Could you check a few things on this drawing? It's one solid part, dimensions in mm from its lowest x, y, z. A direction names the side the tool comes from. Give positions to 0.01 mm unless a question says otherwise; leave off trailing zeros. Order: outer loops, then holes, each group sorted by start corner. A loop starts at its lowest first (then second) coordinate and runs counter-clockwise, first axis right, second up. Notation, with made-up numbers: M 26,1.25 L 82,1.25 A20 ccw 82,11.25 Z; hole C -39,-16 d10. An arc over 180 degrees is marked long. Use one line per item in the form item = value.
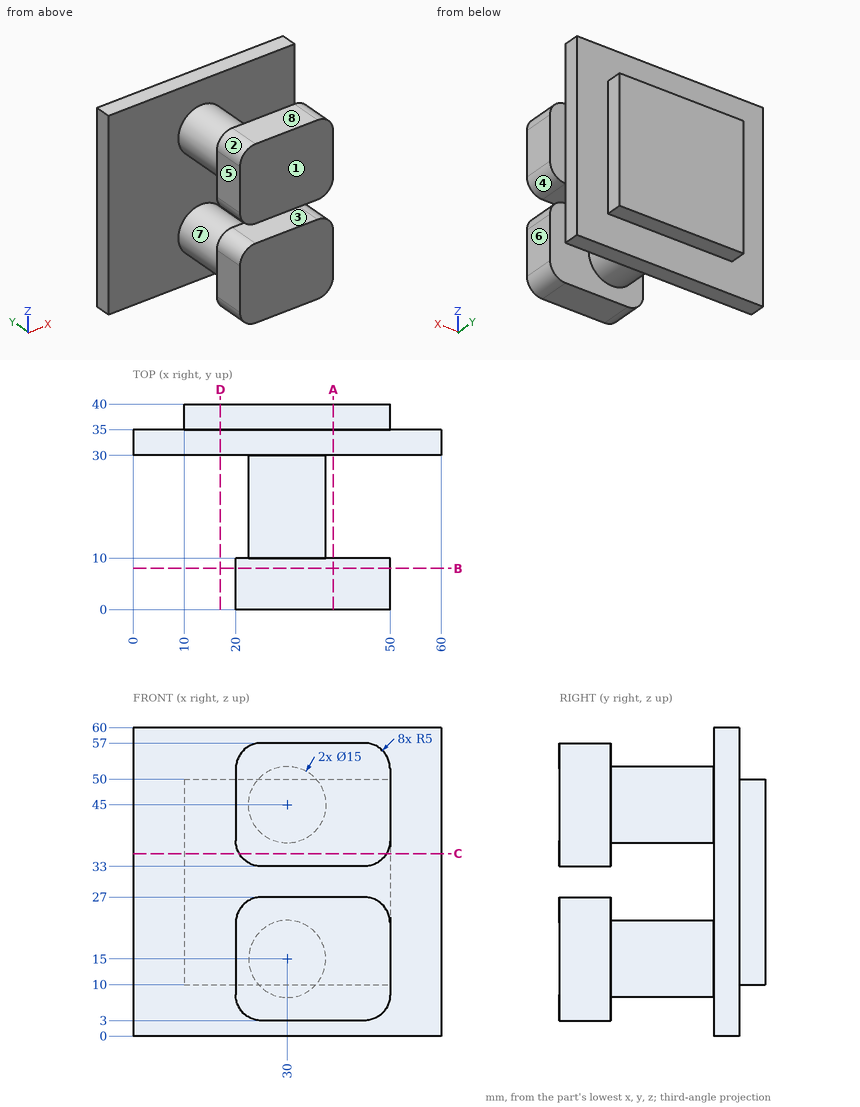
Q1. I want a section at B-B on y = 8. Write out the boundary of the cut face in (x, z), then the cut area to 3 significant figures.
Found:
outline = M 20,8 A5 ccw 25,3 L 45,3 A5 ccw 50,8 L 50,22 A5 ccw 45,27 L 25,27 A5 ccw 20,22 Z; M 20,38 A5 ccw 25,33 L 45,33 A5 ccw 50,38 L 50,52 A5 ccw 45,57 L 25,57 A5 ccw 20,52 Z
area = 1,400 mm²
Q2. I'm going to push flat-ended pins straight in: pin 1 Ø11 at (y, z) = (3.5, 41.5) entering from -X; pin 2 Ø2 at (y, z) = (22.5, 11.5) entering from -X; pin 3 Ø5 at (x, y) = (34, 4.5) entering from +Z. Where does each tip first touch, or does it pass through?
Found:
pin_1 = 20
pin_2 = 22.93
pin_3 = 57
Q3. I want a section at C-C on z = 35.5. Write out the boundary of the cut face in (x, y), then the cut area to 3 significant figures.
Found:
outline = M 0,30 L 60,30 L 60,35 L 50,35 L 50,40 L 10,40 L 10,35 L 0,35 Z; M 20.67,0 L 49.33,0 L 49.33,10 L 20.67,10 Z
area = 787 mm²
Q4. I need wall thicknesses on L1, parallel to Z at x = 44.5, y = 5.5; L2, parallel to Y at x = 42.5, z = 21.5; L3, parallel to Y at x = 43.5, z = 3.5. Which ranges of each line are inside material? Lowest first, please.
Found:
L1 = 3 to 27, 33 to 57
L2 = 0 to 10, 30 to 40
L3 = 0 to 10, 30 to 35
Q5. On a 3-axis mill with a long thin cutter (end or side, diameter ignored), from which of +Z, -Z, +X, -X, +Y, -Y can I reach the whole of each face in a straight line? I mean the marked faces 5, 6, 7 and 8. Say none if no direction works.
Found:
face_5 = +Z, -Z, -X, -Y
face_6 = +Z, -Z, +X, -Y
face_7 = none
face_8 = +Z, +X, -X, -Y
Q6. I want a section at D-D on x = 17. Write out the boundary of the cut face in (y, z), then the cut area to 3 significant figures.
Found:
outline = M 30,0 L 35,0 L 35,10 L 40,10 L 40,50 L 35,50 L 35,60 L 30,60 Z
area = 500 mm²
Q7. I want a section at A-A on x = 39. Write out the boundary of the cut face in (y, z).
Found:
outline = M 0,3 L 10,3 L 10,27 L 0,27 Z; M 0,33 L 10,33 L 10,57 L 0,57 Z; M 30,0 L 35,0 L 35,10 L 40,10 L 40,50 L 35,50 L 35,60 L 30,60 Z
Q8. Thinking about a two-plate mould opening in Z: for the marked faces 1, 2, 3 and 4, which applies, +Z half, -Z half, draft (parallel to the pull), parting line (faces both ways), or undercut?
Found:
face_1 = draft
face_2 = +Z half
face_3 = undercut
face_4 = undercut
